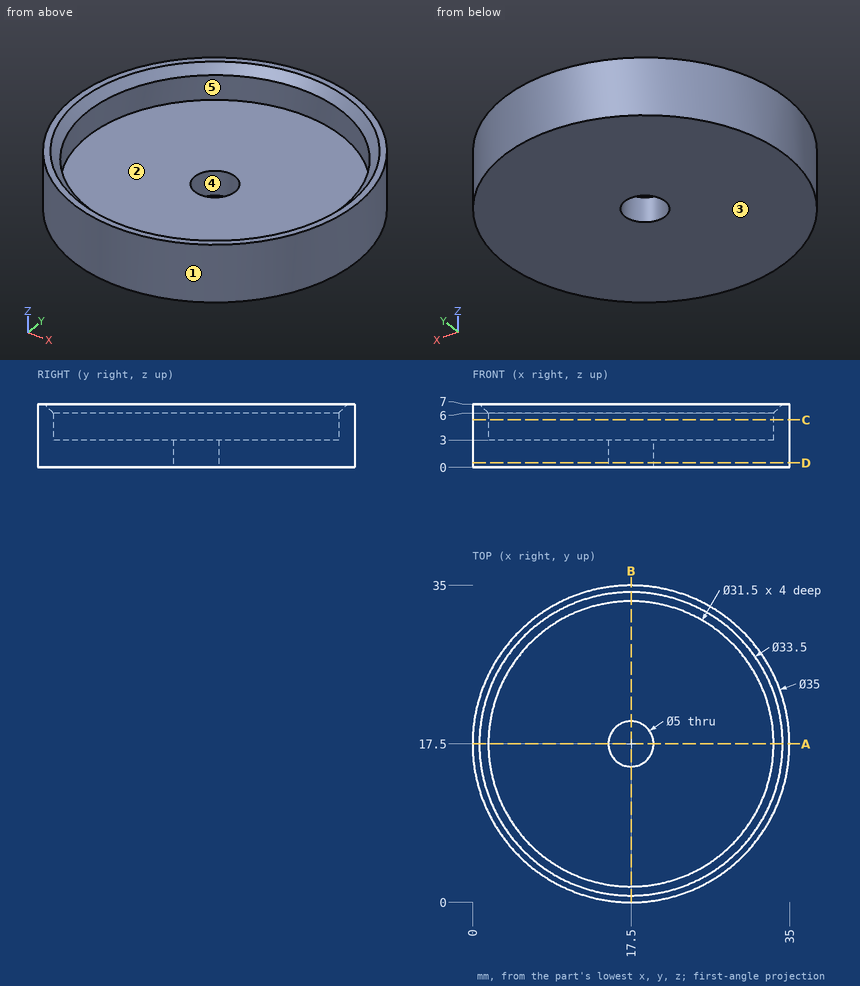
Study the drawing (mm; zero at the part's minimum x, y, z) and answer. A direction names the side the tool comes from. Coordinates: 2 decimals unless noted, no trailing zeros. Write each loop counter-clockwise with the first axis right and the second up, starting at its lowest first coordinate (ties: lowest second). Pieces come first, ordered by that corner, then holes. Notation, with made-up numbers: (23, -9) - (46, -9) arc R22 ccw to (46, 29) - close; hole circle Ø9 at (26, 54.5). An arc over 180 degrees is marked (long way). Answer as a JSON object with one key per item and string values.
Q1. For a pull along Y with two mould halves and no side action, classify the marked faces 1, 2 and 3 as pulls with the +Y half, pulls with the -Y half, needs draft (parallel to the pull), parting line crosses it, or undercut.
Results list:
{"face 1": "parting line crosses it", "face 2": "undercut", "face 3": "needs draft"}
Q2. Which of the six approach directions +Z, -Z, +X, -X, +Y, -Y give full straight-line access (tool end or side, diameter ignored) to the marked faces 4 and 5?
Results list:
{"face 4": "+Z, -Z", "face 5": "+Z"}
Q3. Find section C-C (z = 5.25). Write down the section's boundary in (x, y), plus the area to 3 significant figures.
Results list:
{"outline": "circle Ø35 at (17.5, 17.5); hole circle Ø31.5 at (17.5, 17.5)", "area": "183 mm^2"}
Q4. Find section A-A (y = 17.5). Write down the section's boundary in (x, z).
Results list:
{"outline": "(0, 0) - (15, 0) - (15, 3) - (1.75, 3) - (1.75, 6) - (0.75, 7) - (0, 7) - close; (20, 0) - (35, 0) - (35, 7) - (34.25, 7) - (33.25, 6) - (33.25, 3) - (20, 3) - close"}
Q5. Find section D-D (z = 0.5). Write down the section's boundary in (x, y), plus the area to 3 significant figures.
Results list:
{"outline": "circle Ø35 at (17.5, 17.5); hole circle Ø5 at (17.5, 17.5)", "area": "942 mm^2"}
Q6. Consider L1, parallel to Y at x = 17.5, z = 3.95; L2, parallel to Z at x = 14.5, y = 14; L3, parallel to Y at x = 29, z = 5.25. Determine where each line is inside the solid, lowest interval first. Write a range as from..to.
Results list:
{"L1": "y = 0..1.75, 33.25..35", "L2": "z = 0..3", "L3": "y = 4.31..6.74, 28.26..30.69"}
Q7. Given pin 1 Ø5 at (x, y) = (23, 5) entering from +Z; pin 2 Ø16 at (x, y) = (22, 16.5) entering from +Z; pin 3 Ø1.5 at (x, y) = (12.5, 8) entering from -Z; pin 4 Ø3 at (x, z) = (25, 3) entering from -Y, each flat-ended and moving along its own axis, determine where each tip first touches the part or whether it passes through.
Results list:
{"pin 1": "stops at z = 6.41", "pin 2": "stops at z = 3", "pin 3": "stops at z = 0", "pin 4": "stops at y = 1.06"}
